```python
from build123d import *

# Parameters (mm, degrees)
F0_R      = 38.330172
F1_DEPTH  = 6.9
F2_R      = 27.529056
F3_DEPTH  = 1.8
F4_R      = 29.262122
F5_DEPTH  = 1.1
F8_DEPTH  = 1.5
F6_W      = 12.082048
F6_H      = 33.561243
F9_DEPTH  = 0.6
F10_R     = 4.120832
F11_DEPTH = 25


with BuildPart() as f1:
    # F0 (on Front) → F1 (new body)
    with BuildSketch(Plane.XZ):
        with Locations((-38.259815, 37.991326)):
            Circle(F0_R)
    extrude(amount=F1_DEPTH)

    # F2 (on face) → F3 (cut)
    with BuildSketch(Plane.XZ.offset(6.9)):
        with Locations((-38.259815, 37.991326)):
            Circle(F2_R)
    extrude(amount=-F3_DEPTH, mode=Mode.SUBTRACT)

    # F4 (on face) → F5 (cut)
    with BuildSketch(Plane(origin=(0, 0, 0), x_dir=(-1, 0, 0), z_dir=(0, 1, 0))):
        with Locations((38.259815, 37.991326)):
            Circle(F4_R)
    extrude(amount=-F5_DEPTH, mode=Mode.SUBTRACT)

    # F7 (on face) → F8 (cut)
    with BuildSketch(Plane(origin=(0, -1.1, 0), x_dir=(-1, 0, 0), z_dir=(0, 1, 0))):
        Polygon((44.951111, 56.248643), (32.869063, 56.248643), (32.600574, 23.22438), (44.951111, 23.22438), align=None)
    extrude(amount=-F8_DEPTH, mode=Mode.SUBTRACT)

    # F6 (on face) → F9 (cut)
    with BuildSketch(Plane.XZ.offset(5.1)):
        with Locations((-38.931042, 39.468021)):
            Rectangle(F6_W, F6_H)
    extrude(amount=-F9_DEPTH, mode=Mode.SUBTRACT)

    # F10 (on face) → F11 (cut)
    with BuildSketch(Plane.XZ.offset(6.9)):
        with Locations((-17.46659, 64.012818)):
            Circle(F10_R)
    extrude(amount=-F11_DEPTH, mode=Mode.SUBTRACT)


solid = f1.part
```
Geometry check sheet. Reference: the model listing, model coordinates, mm. A direction names the side the tool comes from. Coordinates: 2 decimals unless noted, no trailing zeros. Order: outer loops, then holes, each group sorted by start corner. A loop starts at its lowest first (then second) coordinate and runs counter-clockwise, first axis right, second up.
Q1. Sectioned sample at A-A on x = -18. Record the cut outline in (y, z).
Reply:
outline: (-6.9, 5.45) - (0, 5.45) - (0, 16.88) - (-1.1, 16.88) - (-1.1, 59.11) - (0, 59.11) - (0, 59.93) - (-6.9, 59.93) - (-6.9, 56.63) - (-5.1, 56.63) - (-5.1, 19.35) - (-6.9, 19.35) - close; (-6.9, 68.1) - (0, 68.1) - (0, 70.53) - (-6.9, 70.53) - close
Q2. Depth check by flat-ended pin: pin 1 Ø1.5 at (y, z) = (-3, 67) entering from -X; pin 2 Ø4 at (y, z) = (-4.5, 51.5) entering from +X; pin 3 Ø3.5 at (x, z) = (-36, 40) entering from -Y. Enter the tip coordinate at first touch or a pass-through.
Reply:
pin 1: stops at x = -64.16
pin 2: stops at x = -1.7
pin 3: stops at y = -4.5
Q3. Sectioned sample at B-B on z = 12.5. Record the cut outline in (x, y).
Reply:
outline: (-66.88, -6.9) - (-48.65, -6.9) - (-48.65, -5.1) - (-27.87, -5.1) - (-27.87, -6.9) - (-9.63, -6.9) - (-9.63, 0) - (-23.89, 0) - (-23.89, -1.1) - (-52.63, -1.1) - (-52.63, 0) - (-66.88, 0) - close
Q4. Sectioned sample at C-C on x = -28.5. Record the cut outline in (y, z), and give its area (3 significant figures).
Reply:
outline: (-6.9, 0.92) - (0, 0.92) - (0, 10.4) - (-1.1, 10.4) - (-1.1, 65.58) - (0, 65.58) - (0, 75.06) - (-6.9, 75.06) - (-6.9, 63.73) - (-5.1, 63.73) - (-5.1, 12.25) - (-6.9, 12.25) - close
area: 358 mm2
Q5. Tool access check on faces 1 (the face through (-31, -1.1, 38)), 2 (the face through (-15.565, -3.498, 60.357)), 3 (the face through (-41.844, -6.013, 65.286)). Record the directions out of +Z, -Z, +X, -X, +Y, -Y that give a thin tool (end or side, any length) a straight path to the whole face; none if there is none.
Reply:
face 1: +Y
face 2: +Y, -Y
face 3: -Y
Q6. Thickness scan on probe 1 along Z at (x, y) = (-39, -5.75); probe 2 along Y at (x, z) = (-11.5, 42); probe 3 along X at (y, z) = (-6.25, 63.5). Record the ranges inside material, lowest first.
Reply:
probe 1: z = -0.33 to 10.47, 65.51 to 76.31
probe 2: y = -5.1 to -1.1
probe 3: x = -66.87 to -48.61, -27.91 to -21.56, -13.38 to -9.65
Q7. Draft check along Z on faces 4 (the face through (-47, 0, 9.8)), 5 (the face through (-20.573, -3.402, 3.986)), 6 (the face through (-32.5, -5.1, 38.4)). Enter one of: released by +Z, released by -Z, zero draft, split by the parting line, or undercut.
Reply:
face 4: zero draft
face 5: split by the parting line
face 6: undercut
Q8. Sectioned sample at D-D on y = -3.5. Record the cut outline in (x, z).
Reply:
outline: circle Ø76.66 at (-38.26, 37.99); hole circle Ø8.24 at (-17.47, 64.01)
